from build123d import *

# Parameters (mm, degrees)
F1_DEPTH = 152.4
F2_R     = 3.81
F3_R     = 2.54


with BuildPart() as f1:
    # F0 (on Front) → F1 (new body)
    with BuildSketch(Plane.XZ):
        Polygon((0, 25.4), (0, 0), (25.4, 0), align=None)
    extrude(amount=F1_DEPTH)

    # F2
    f2_edges = [f1.edges().sort_by_distance(p)[0] for p in [
        (0, -76.2, 25.4),
        (25.4, -76.2, 0),
    ]]
    fillet(f2_edges, radius=F2_R)

    # F3
    f3_edges = [f1.edges().sort_by_distance(p)[0] for p in [
        (0, -76.2, 0),
    ]]
    fillet(f3_edges, radius=F3_R)


solid = f1.part
Model file for the job. Use its own axes, mm. Round coordinates to 2 decimals unless told otherwise and drop trailing zeros. Loops run counter-clockwise (first coordinate to the right, second up) from the corner with the lowest first, then second, coordinate; pieces in that order, holes last.
1. Wall check: probe 1 along Z at (x, y) = (11, -127.5); probe 2 along Z at (x, y) = (13.75, -43); probe 3 along X at (y, z) = (-110, 18.75). Give the ranges that are in metal, low to high.
Check values:
probe 1: z = 0 to 14.4
probe 2: z = 0 to 11.65
probe 3: x = 0.98 to 6.65
2. Band-saw the part on B-B, the plane x = 12.25. List the corners of the cut face in (y, z), and give its area (3 significant figures).
Check values:
outline: (-152.4, 0) - (0, 0) - (0, 13.15) - (-152.4, 13.15) - close
area: 2,000 mm2
3. Band-saw the part on A-A, the plane y = -46. List the corners of the cut face in (x, z).
Check values:
outline: (0, 2.54) arc R2.54 ccw to (2.54, 0) - (16.2, 0) arc R3.81 ccw to (18.9, 6.5) - (6.5, 18.9) arc R3.81 ccw to (0, 16.2) - close
4. Drop flat-ended pins along their axis: P1, Ø6, axis at y = -55, z = 12.5, coming from the +X side; P2, Ø1.5, axis at x = 17.5, y = -126.5, coming from the -Z side; P3, Ø4, axis at x = 15, y = -131, coming from the +Z side. Give the stop position or say it passes through.
Check values:
P1: stops at x = 15.9
P2: stops at z = 0.04
P3: stops at z = 12.4
5. Band-saw the part on C-C, the plane z = 14. List the corners of the cut face in (x, y).
Check values:
outline: (0, -152.4) - (11.4, -152.4) - (11.4, 0) - (0, 0) - close
